from build123d import *

# Parameters (mm, degrees)
SKETCH1_R           = 81
SKETCH1_R_2         = 1.55
SKETCH1_R_3         = 12
BOSS_EXTRUDE1_DEPTH = 2
CUT_EXTRUDE1_DEPTH  = 5


with BuildPart() as part:
    # Sketch1 → Boss-Extrude1 (new body, symmetric)
    with BuildSketch(Plane(origin=(0, 0, 0), x_dir=(1, 0, 0), z_dir=(0, 1, 0))):
        Circle(SKETCH1_R)
        with Locations((43.301270189, 25)):
            Circle(SKETCH1_R_2, mode=Mode.SUBTRACT)
        with Locations((0, -50)):
            Circle(SKETCH1_R_2, mode=Mode.SUBTRACT)
        with Locations((-43.301270189, 25)):
            Circle(SKETCH1_R_2, mode=Mode.SUBTRACT)
        Circle(SKETCH1_R_3, mode=Mode.SUBTRACT)
    extrude(amount=BOSS_EXTRUDE1_DEPTH, both=True)

    # Sketch2 → Cut-Extrude1 (cut, through all)
    with BuildSketch(Plane.XZ.offset(2)):
        with BuildLine():
            ThreePointArc((-66.704830818, -45.950686018), (-58.889727457, -34), (-73.146876822, -34.792735035))
            ThreePointArc((-73.146876822, -34.792735035), (-70.148057707, -40.5), (-66.704830818, -45.950686018))
        make_face()
        with BuildLine():
            ThreePointArc((66.704830818, -45.950686018), (70.148057707, -40.5), (73.146876822, -34.792735035))
            ThreePointArc((73.146876822, -34.792735035), (58.889727457, -34), (66.704830818, -45.950686018))
        make_face()
        with BuildLine():
            ThreePointArc((-6.442046004, 80.743421053), (0, 68), (6.442046004, 80.743421053))
            ThreePointArc((6.442046004, 80.743421053), (0, 81), (-6.442046004, 80.743421053))
        make_face()
    extrude(amount=-CUT_EXTRUDE1_DEPTH, mode=Mode.SUBTRACT)


solid = part.part
Geometry check sheet. Reference: the model listing, model coordinates, mm. Give positions to 0.01 mm unless a question says otherwise; leave off trailing zeros. Write each loop counter-clockwise with the first axis right and the second up, starting at its lowest first coordinate (ties: lowest second). Pieces come first, ordered by that corner, then holes. Notation, with made-up numbers: M 63,75 L 78,75 A22 ccw 78,88 Z; hole C -6.75,51.25 d1. An arc over 180 degrees is marked long. Answer as CSV lines item,"result". Start each with the question number.
Q1. Go/stop test with flat-tipped pins: pin 1 (1 mm diameter, centred on y = -0.5, z = -13, fed in from -X); pin 2 (1.5 mm diameter, centred on y = 1, z = 30.5, fed in from -X). Record where each tip stops, or that it passes through.
Q2. Material ranges on L1, parallel to X at y = 1.25, z = -25; L2, parallel to X at y = -0.4, z = -7.5; L3, parallel to X at y = 0.9, z = -0.5, recorded low to high.
Q3. Section check D-D, the plane x = 28. Record the cut outline in (y, z).
Q4. Section check C-C, the plane z = 76. Record the cut outline in (x, y), then the cut area to 3 significant figures.
Q5. Section check B-B, the plane y = -1.05. Record the cut outline in (x, z).
Q6. Section check A-A, the plane z = 0. Record the cut outline in (x, y), then the cut area to 3 significant figures.
Q7. Release check for a two-part mould opening along Z. For faces 1 (the face through (-1, -2, 17)), 2 (the face through (69.59, 0.03, 41.45)), 3 (the face through (59.017, -0.028, -33.788)) record: pulls with the +Z half, pulls with the -Z half, needs draft (parallel to the pull), parting line crosses it, or undercut.
Geometry says:
1,pin 1,"x = -80.03"
1,pin 2,"x = -75.34"
2,L1,"-77.05 to -44.85, -41.75 to 41.75, 44.85 to 77.05"
2,L2,"-80.65 to -9.37, 9.37 to 80.65"
2,L3,"-81 to -11.99, 11.99 to 81"
3,outline,"M -2,-76.01 L 2,-76.01 L 2,76.01 L -2,76.01 Z"
4,outline,"M -28.02,-2 L -8,-2 L -8,2 L -28.02,2 Z; M 8,-2 L 28.02,-2 L 28.02,2 L 8,2 Z"
4,area,"160 mm^2"
5,outline,"M -73.15,-34.79 A8 cw long -66.7,-45.95 A81 ccw 66.7,-45.95 A8 cw long 73.15,-34.79 A81 ccw 6.44,80.74 A8 cw long -6.44,80.74 A81 ccw Z; hole C -43.3,-25 d3.1; hole C 0,0 d24; hole C 0,50 d3.1; hole C 43.3,-25 d3.1"
6,outline,"M -81,-2 L -12,-2 L -12,2 L -81,2 Z; M 12,-2 L 81,-2 L 81,2 L 12,2 Z"
6,area,"552 mm^2"
7,face 1,"needs draft"
7,face 2,"parting line crosses it"
7,face 3,"undercut"
